Work out the finished part from the listing and answer in its coordinate system (mm). Round coordinates to 2 decimals unless told otherwise and drop trailing zeros. Loops run counter-clockwise (first coordinate to the right, second up) from the corner with the lowest first, then second, coordinate; pieces in that order, holes last. Notation, with made-up numbers: M -4,39 L 6,39 A21 cw 6,71 Z; hole C 31,-12 d7. An arc over 180 degrees is marked long. One line per item, written item: value.
```python
from build123d import *

# Parameters (mm, degrees)
F0_W           = 106
F0_H           = 65
F0_R           = 2
F1_DEPTH       = 3
F3_D           = 3
F3_CSINK_D     = 6.72
F3_CSINK_ANGLE = 82
F4_R           = 5


with BuildPart() as f1:
    # F0 (on Top) → F1 (new body)
    with BuildSketch(Plane.XY):
        with Locations((53, 32.5)):
            Rectangle(F0_W, F0_H)
        with Locations((5, 5)):
            Circle(F0_R, mode=Mode.SUBTRACT)
        with Locations((101, 5)):
            Circle(F0_R, mode=Mode.SUBTRACT)
        with Locations((5, 60)):
            Circle(F0_R, mode=Mode.SUBTRACT)
        with Locations((101, 60)):
            Circle(F0_R, mode=Mode.SUBTRACT)
    extrude(amount=F1_DEPTH)

    # F3 (through all)
    with Locations(Plane.XY.offset(3)):
        with Locations((53, 39), (53, 26)):
            CounterSinkHole(F3_D / 2, F3_CSINK_D / 2, counter_sink_angle=F3_CSINK_ANGLE)

    # F4
    f4_edges = [f1.edges().sort_by_distance(p)[0] for p in [
        (106, 0, 1.5),
        (0, 0, 1.5),
        (0, 65, 1.5),
        (106, 65, 1.5),
    ]]
    fillet(f4_edges, radius=F4_R)


solid = f1.part
```
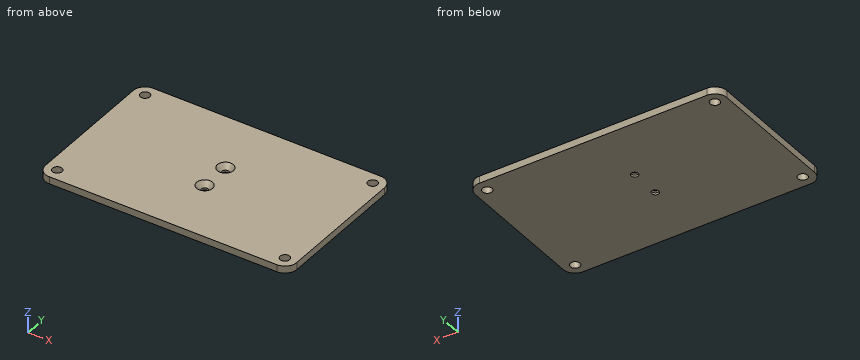
1) Each of these flat-tipped pins is pushed along its axis until it touches: pin 1 (5 mm diameter, centred on x = 53, y = 26, fed in from +Z); pin 2 (4 mm diameter, centred on x = 53, y = 39, fed in from +Z); pin 3 (5 mm diameter, centred on x = 72.5, y = 9, fed in from -Z); pin 4 (2.5 mm diameter, centred on x = 5, y = 60, fed in from -Z). Where does it stop, or does it pass through?
Check values:
pin 1: z = 2.01
pin 2: z = 1.44
pin 3: z = 0
pin 4: through
2) Find section A-A (x = 53). Give the vertices of the cut face in (y, z), then the cut area to 3 significant figures.
Check values:
outline: M 0,0 L 24.5,0 L 24.5,0.86 L 22.64,3 L 0,3 Z; M 27.5,0 L 37.5,0 L 37.5,0.86 L 35.64,3 L 29.36,3 L 27.5,0.86 Z; M 40.5,0 L 65,0 L 65,3 L 42.36,3 L 40.5,0.86 Z
area: 169 mm2
3) Find the intervals of material crossed by probe 1 along Y at (x, z) = (5, 1.5); probe 2 along X at (y, z) = (39, 0.45); probe 3 along Y at (x, z) = (6.5, 0.85), in increasing order. Write a range as from..to.
Check values:
probe 1: 0..3, 7..58, 62..65
probe 2: 0..51.5, 54.5..106
probe 3: 0..3.68, 6.32..58.68, 61.32..65
